```python
from build123d import *

# Parameters (mm, degrees)
ESQUISSE1_W             = 163
ESQUISSE1_H             = 120
BOSS_EXTRU_1_DEPTH      = 1.5
CONG_2_R                = 6.5
ESQUISSE4_R             = 2.5
ENL_V_MAT_EXTRU_3_DEPTH = 174.698733444
ESQUISSE7_R             = 1.5
ENL_V_MAT_EXTRU_5_DEPTH = 174.698733444
ESQUISSE8_R             = 8.1
ENL_V_MAT_EXTRU_6_DEPTH = 174.698733444
ESQUISSE9_R             = 1.5
ENL_V_MAT_EXTRU_7_DEPTH = 174.698733444


with BuildPart() as part:
    # Esquisse1 → Boss.-Extru.1 (new body)
    with BuildSketch(Plane(origin=(0, 0, 0), x_dir=(1, 0, 0), z_dir=(0, 1, 0))):
        with Locations((81.5, 0)):
            Rectangle(ESQUISSE1_W, ESQUISSE1_H)
    extrude(amount=BOSS_EXTRU_1_DEPTH)

    # Congé2
    cong_2_edges = [part.edges().sort_by_distance(p)[0] for p in [
        (163, 0.75, -60),
        (163, 0.75, 60),
    ]]
    fillet(cong_2_edges, radius=CONG_2_R)

    # Esquisse4 → Enlèv. mat.-Extru.3 (cut, through all)
    with BuildSketch(Plane(origin=(0, 1.5, 0), x_dir=(1, 0, 0), z_dir=(0, 1, 0))):
        with Locations(Location((120, -50, 0), (0, 0, 270))):
            Circle(ESQUISSE4_R)
        with Locations(Location((38, -50, 0), (0, 0, 270))):
            Circle(ESQUISSE4_R)
        with Locations(Location((38, 50, 0), (0, 0, 90))):
            Circle(ESQUISSE4_R)
        with Locations(Location((120, 50, 0), (0, 0, 90))):
            Circle(ESQUISSE4_R)
    extrude(amount=-ENL_V_MAT_EXTRU_3_DEPTH, mode=Mode.SUBTRACT)

    # Symétrie1: part across plane


with BuildPart() as part_1:
    add(part.part)
    add(part.part.mirror(Plane(origin=(0, 1.5, -60), x_dir=(0, 0, 1), z_dir=(1, 0, 0))))

    # Esquisse7 → Enlèv. mat.-Extru.5 (cut, through all)
    with BuildSketch(Plane(origin=(0, 1.5, 0), x_dir=(1, 0, 0), z_dir=(0, 1, 0))):
        with Locations(Location((-156, -51, 0), (0, 0, 270))):
            Circle(ESQUISSE7_R)
        with Locations(Location((-104, -51, 0), (0, 0, 270))):
            Circle(ESQUISSE7_R)
        with Locations(Location((-52, -51, 0), (0, 0, 270))):
            Circle(ESQUISSE7_R)
        with Locations(Location((0, -51, 0), (0, 0, 270))):
            Circle(ESQUISSE7_R)
        with Locations(Location((52, -51, 0), (0, 0, 270))):
            Circle(ESQUISSE7_R)
        with Locations(Location((-104, -17, 0), (0, 0, 270))):
            Circle(ESQUISSE7_R)
        with Locations(Location((-52, -17, 0), (0, 0, 270))):
            Circle(ESQUISSE7_R)
        with Locations(Location((0, -17, 0), (0, 0, 270))):
            Circle(ESQUISSE7_R)
        with Locations(Location((52, -17, 0), (0, 0, 270))):
            Circle(ESQUISSE7_R)
        with Locations(Location((-104, 17, 0), (0, 0, 270))):
            Circle(ESQUISSE7_R)
        with Locations(Location((-52, 17, 0), (0, 0, 270))):
            Circle(ESQUISSE7_R)
        with Locations(Location((0, 17, 0), (0, 0, 270))):
            Circle(ESQUISSE7_R)
        with Locations(Location((52, 17, 0), (0, 0, 270))):
            Circle(ESQUISSE7_R)
        with Locations(Location((-156, -17, 0), (0, 0, 270))):
            Circle(ESQUISSE7_R)
        with Locations(Location((-156, 17, 0), (0, 0, 270))):
            Circle(ESQUISSE7_R)
        with Locations(Location((-156, 51, 0), (0, 0, 270))):
            Circle(ESQUISSE7_R)
        with Locations(Location((-104, 51, 0), (0, 0, 270))):
            Circle(ESQUISSE7_R)
        with Locations(Location((-52, 51, 0), (0, 0, 270))):
            Circle(ESQUISSE7_R)
        with Locations(Location((0, 51, 0), (0, 0, 270))):
            Circle(ESQUISSE7_R)
        with Locations(Location((52, 51, 0), (0, 0, 270))):
            Circle(ESQUISSE7_R)
        with Locations(Location((104, -51, 0), (0, 0, 270))):
            Circle(ESQUISSE7_R)
        with Locations(Location((104, -17, 0), (0, 0, 270))):
            Circle(ESQUISSE7_R)
        with Locations(Location((104, 17, 0), (0, 0, 270))):
            Circle(ESQUISSE7_R)
        with Locations(Location((104, 51, 0), (0, 0, 270))):
            Circle(ESQUISSE7_R)
        with Locations(Location((156, -51, 0), (0, 0, 270))):
            Circle(ESQUISSE7_R)
        with Locations(Location((156, -17, 0), (0, 0, 270))):
            Circle(ESQUISSE7_R)
        with Locations(Location((156, 17, 0), (0, 0, 270))):
            Circle(ESQUISSE7_R)
        with Locations(Location((156, 51, 0), (0, 0, 270))):
            Circle(ESQUISSE7_R)
    extrude(amount=-ENL_V_MAT_EXTRU_5_DEPTH, mode=Mode.SUBTRACT)

    # Esquisse8 → Enlèv. mat.-Extru.6 (cut, through all)
    with BuildSketch(Plane(origin=(0, 1.5, 0), x_dir=(1, 0, 0), z_dir=(0, 1, 0))):
        with Locations(Location((0, 0, 0), (0, 0, 270))):
            Circle(ESQUISSE8_R)
        with Locations(Location((-78, 0, 0), (0, 0, 270))):
            Circle(ESQUISSE8_R)
        with Locations(Location((78, 0, 0), (0, 0, 270))):
            Circle(ESQUISSE8_R)
    extrude(amount=-ENL_V_MAT_EXTRU_6_DEPTH, mode=Mode.SUBTRACT)

    # Esquisse9 → Enlèv. mat.-Extru.7 (cut, through all)
    with BuildSketch(Plane(origin=(0, 1.5, 0), x_dir=(1, 0, 0), z_dir=(0, 1, 0))):
        with Locations(Location((27.5, 32.5, 0), (0, 0, 270))):
            Circle(ESQUISSE9_R)
        with Locations(Location((-13, -30, 0), (0, 0, 270))):
            Circle(ESQUISSE9_R)
        with Locations(Location((35, -20, 0), (0, 0, 270))):
            Circle(ESQUISSE9_R)
        with Locations(Location((-27.5, 32.5, 0), (0, 0, 90))):
            Circle(ESQUISSE9_R)
    extrude(amount=-ENL_V_MAT_EXTRU_7_DEPTH, mode=Mode.SUBTRACT)


solid = part_1.part
```
CAD build for the part. Positions are in the model's coordinates, mm. Round coordinates to 2 decimals unless told otherwise and drop trailing zeros. Order: outer loops, then holes, each group sorted by start corner. A loop starts at its lowest first (then second) coordinate and runs counter-clockwise, first axis right, second up. Notation, with made-up numbers: (82.25, 78) -> (86.25, 78) arc R23 cw to (86.25, 93) -> close; hole circle Ø4 at (8.5, -33). An arc over 180 degrees is marked (long way). Write item = value, one per line.
(1) Cut at B-B (y = 0.3). State how many separate pieces and enclosed holes the cut face has, plus the area to 3 significant figures.
Answers follow:
separate_pieces = 1
enclosed_holes = 43
area = 38,100 mm²
(2) Pull direction Z, two halves, no side cores. Call faces 1 (the flat face through (2, 0, -14)), 2 (the cylindrical face through (-161.045, 0.76, 58.146)), 3 (the cylindrical face through (-69.97, 0.76, -1.05)): +Z half, -Z half, draft (parallel to the pull), parting line (faces both ways), or undercut.
Answers follow:
face_1 = draft
face_2 = +Z half
face_3 = undercut
(3) Flat gauge pin, fed straight in: P1, Ø2.5, axis at x = -104, z = -17, coming from the +Y side. Where does the tip first touch, or does it go through?
Answers follow:
P1 = through
(4) Cut at A-A (x = -78). Write the cut outline in (y, z), plus the area to 3 significant figures.
Answers follow:
outline = (0, -60) -> (1.5, -60) -> (1.5, -8.1) -> (0, -8.1) -> close; (0, 8.1) -> (1.5, 8.1) -> (1.5, 60) -> (0, 60) -> close
area = 156 mm²
(5) Drill centre lines: L1, parallel to X at y = 1.3, z = 0; L2, parallel to Z at x = -120, y = 0.8; L3, parallel to X at y = 1.4, z = -1.5. Where is each one in solid material? Low to high.
Answers follow:
L1 = -163 to -86.1, -69.9 to -8.1, 8.1 to 69.9, 86.1 to 163
L2 = -60 to -52.5, -47.5 to 47.5, 52.5 to 60
L3 = -163 to -85.96, -70.04 to -7.96, 7.96 to 70.04, 85.96 to 163
